Source: CAD feature listing. Evaluate the final solid. Frame: model axes, mm. A direction names the side the tool comes from. Coordinates: 2 decimals unless noted, no trailing zeros. Loops run counter-clockwise (first coordinate to the right, second up) from the corner with the lowest first, then second, coordinate; pieces in that order, holes last. Notation, with made-up numbers: M 5,70 L 46,70 A22 ccw 46,104 Z; hole C 65,56.5 d9. An arc over 180 degrees is marked long. Write each question's results on one line, items separated by ' | '. Start each with the question number.
from build123d import *

# Parameters (mm, degrees)
SKETCH1_W           = 40
SKETCH1_H           = 40
BOSS_EXTRUDE1_DEPTH = 20
CHAMFER1_SIZE       = 20
SKETCH2_W           = 3
SKETCH2_H           = 5
SKETCH2_W_2         = 5
SKETCH2_H_2         = 3
CUT_EXTRUDE1_DEPTH  = 20
SKETCH3_W           = 17.5
SKETCH3_H           = 3
SKETCH3_W_2         = 3
SKETCH3_H_2         = 17.5
SKETCH3_H_3         = 7.5
SKETCH3_W_3         = 7.5
BOSS_EXTRUDE2_DEPTH = 8
SKETCH4_R           = 1.5
BOSS_EXTRUDE3_DEPTH = 5
SKETCH6_R           = 1.5
BOSS_EXTRUDE4_DEPTH = 5


with BuildPart() as part:
    # Sketch1 → Boss-Extrude1 (new body)
    with BuildSketch(Plane(origin=(0, 0, 0), x_dir=(1, 0, 0), z_dir=(0, 1, 0))):
        with Locations((-1.65921027, -4.12371134)):
            Rectangle(SKETCH1_W, SKETCH1_H)
    extrude(amount=BOSS_EXTRUDE1_DEPTH)

    # Chamfer1
    chamfer1_edges = [part.edges().sort_by_distance(p)[0] for p in [
        (18.34078973, 20, 4.12371134),
        (-1.65921027, 20, 24.12371134),
    ]]
    chamfer(chamfer1_edges, length=CHAMFER1_SIZE - 0.0001)  # a hair under: the kernel refuses the full size

    # Sketch2 → Cut-Extrude1 (cut)
    with BuildSketch(Plane.XZ):
        Polygon((15.34078973, 21.12371134), (15.34078973, 14.12371134), (18.34078973, 14.12371134), (18.34078973, 24.12371134), (8.34078973, 24.12371134), (8.34078973, 21.12371134), align=None)
        with Locations((16.84078973, -5.87628866)):
            Rectangle(SKETCH2_W, SKETCH2_H)
        with Locations((-11.65921027, 22.62371134)):
            Rectangle(SKETCH2_W_2, SKETCH2_H_2)
    extrude(amount=-CUT_EXTRUDE1_DEPTH, mode=Mode.SUBTRACT)

    # Sketch3 → Boss-Extrude2 (add)
    with BuildSketch(Plane.XZ):
        with Locations((-0.40921027, 22.62371134)):
            Rectangle(SKETCH3_W, SKETCH3_H)
        with Locations((16.84078973, 5.37371134)):
            Rectangle(SKETCH3_W_2, SKETCH3_H_2)
        with Locations((16.84078973, -12.12628866)):
            Rectangle(SKETCH3_W_2, SKETCH3_H_3)
        with Locations((-17.90921027, 22.62371134)):
            Rectangle(SKETCH3_W_3, SKETCH3_H)
    extrude(amount=BOSS_EXTRUDE2_DEPTH)

    # Sketch4 → Boss-Extrude3 (add)
    with BuildSketch(Plane.XY.offset(21.12371134)):
        with Locations(Location((-11.65921027, 1.5, 0), (0, 0, 270))):
            Circle(SKETCH4_R)
    extrude(amount=BOSS_EXTRUDE3_DEPTH)

    # Sketch5 → Revolve1 (revolve)
    with BuildSketch(Plane.XY.offset(26.12371134)):
        with BuildLine():
            Line((-11.65921027, 3.5), (-11.65921027, -0.5))
            ThreePointArc((-11.65921027, -0.5), (-9.65921027, 1.5), (-11.65921027, 3.5))
        make_face()
    revolve(axis=Axis((-11.65921027, 3.5, 26.12371134), (0, -1, 0)))

    # Sketch6 → Boss-Extrude4 (add)
    with BuildSketch(Plane(origin=(15.34078973, 0, 0), x_dir=(0, 0, -1), z_dir=(1, 0, 0))):
        with Locations(Location((5.87628866, 1.5, 0), (0, 0, 270))):
            Circle(SKETCH6_R)
    extrude(amount=BOSS_EXTRUDE4_DEPTH)

    # Sketch7 → Revolve2 (revolve)
    with BuildSketch(Plane(origin=(20.34078973, 0, 0), x_dir=(0, 0, -1), z_dir=(1, 0, 0))):
        with BuildLine():
            Line((5.87628866, 3.5), (5.87628866, -0.5))
            ThreePointArc((5.87628866, -0.5), (3.87628866, 1.5), (5.87628866, 3.5))
        make_face()
    revolve(axis=Axis((20.34078973, 3.5, -5.87628866), (0, -1, 0)))


solid = part.part
Item 1: Line query: probe 1 along Y at (x, z) = (-16.5, 2); probe 2 along X at (y, z) = (3, 11); probe 3 along Z at (x, y) = (-1.5, -5.5). Output: solid intervals per line, ascending.
Item 2: First-contact query: pin 1 Ø8 at (y, z) = (14, -2) entering from +X; pin 2 Ø1.5 at (x, y) = (6.5, -1.5) entering from +Z; pin 3 Ø0.9 at (x, y) = (12, 2) entering from +Z. Flat tips, straight axial feed; report the tip coordinate or a pass-through.
Item 3: Cut plane D-D (y = 1). Output: boundary loops of the cut face in (x, z) (1 decimal).
Item 4: Mould query, pull axis X, two halves, no side actions, for faces 1 (the flat face through (18.341, -4, 5)), 2 (the flat face through (-9.159, -4, 23)), 3 (the flat face through (-3, 0, 2)). Classes: +X half, -X half, draft (parallel to the pull), parting line (faces both ways), or undercut.
Item 5: Access query for faces 4 (the flat face through (-1, -4, 21.124)), 5 (the cylindrical face through (17.154, 2.606, -6.89)), 6 (the flat face through (17, -4, 14.124)). Directions: +Z, -Z, +X, -X, +Y, -Y. A direction counts if a zero-diameter tool reaches every point of the face in a straight line with its end or side. Return the directions, or none.
Item 6: Cut plane C-C (x = -16). Output: boundary loops of the cut face in (y, z).
Item 7: Cut plane A-A (y = -4.5). Output: boundary loops of the cut face in (x, z).
Item 8: Cut plane B-B (z = 1). Output: boundary loops of the cut face in (x, y), then the cut area to 3 significant figures.
Response values:
1) probe 1: y = 0 to 20 | probe 2: x = -21.66 to 15.34 | probe 3: z = 21.12 to 24.12
2) pin 1: stops at x = 8.34 | pin 2: stops at z = 24.12 | pin 3: stops at z = 21.12
3) outline: M -21.7,-15.9 L 17.3,-15.9 L 17.3,-8.4 L 15.3,-8.4 L 15.3,-7.3 L 19,-7.3 A1.9 ccw long 19,-4.5 L 15.3,-4.5 L 15.3,-3.4 L 17.3,-3.4 L 17.3,14.1 L 15.3,14.1 L 15.3,21.1 L 8.3,21.1 L 8.3,23.1 L -9.2,23.1 L -9.2,21.1 L -10.2,21.1 L -10.2,24.8 A1.9 ccw long -13.1,24.8 L -13.1,21.1 L -14.2,21.1 L -14.2,23.1 L -21.7,23.1 Z
4) face 1: +X half | face 2: undercut | face 3: draft
5) face 4: -Z, +X, -X, -Y | face 5: none | face 6: +Z, +X, +Y, -Y
6) outline: M -8,21.12 L 0,21.12 L 0,-15.88 L 20,-15.88 L 20,4.12 L 0,24.12 L -8,24.12 Z
7) outline: M -21.66,21.12 L -14.16,21.12 L -14.16,24.12 L -21.66,24.12 Z; M -9.16,21.12 L 8.34,21.12 L 8.34,24.12 L -9.16,24.12 Z; M 15.34,-15.88 L 18.34,-15.88 L 18.34,-8.38 L 15.34,-8.38 Z; M 15.34,-3.38 L 18.34,-3.38 L 18.34,14.12 L 15.34,14.12 Z
8) outline: M -21.66,0 L 15.34,0 L 15.34,-8 L 18.34,-8 L 18.34,0 L -1.66,20 L -21.66,20 Z | area: 624 mm2
